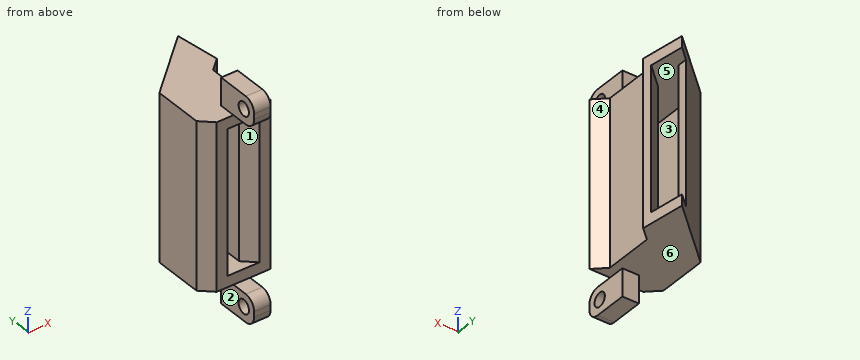
```python
from build123d import *

# Parameters (mm, degrees)
PAD007_DEPTH    = 30
SKETCH021_W     = 5.75
SKETCH021_H     = 26
SKETCH023_W     = 2.875
SKETCH023_H     = 26
POCKET009_DEPTH = 5
SKETCH024_W     = 3
SKETCH024_H     = 3
PAD008_DEPTH    = 5
PAD008_FACE6_W  = 3
PAD008_FACE6_H  = 5
PAD009_DEPTH    = 5
SKETCH025_W     = 3
SKETCH025_H     = 3
PAD010_DEPTH    = 5
PAD010_FACE7_W  = 3
PAD010_FACE7_H  = 5
PAD011_DEPTH    = 5
SKETCH026_R     = 1.25
POCKET010_DEPTH = 5
FILLET_R        = 2


with BuildPart() as part:
    # Sketch020 → Pad007 (new body)
    with BuildSketch(Plane.XY):
        Polygon((-9.75, -21), (-11.9217087917, -19), (-11.9217087917, -10), (-1.063164833, 0), (0, -8), (-2.1717087917, -10), (-2.1717087917, -19), (0, -21), align=None)
    extrude(amount=PAD007_DEPTH)

    # SubtractivePipe: sweep along a path in Sketch022
    with BuildLine(Plane.XY.offset(30)) as subtractivepipe_path:
        Line((-4.875, -21), (-7.0467087917, -19))
        Line((-7.0467087917, -19), (-7.0467087917, -10))
        Line((-7.0467087917, -10), (-0.5315824165, -4))
    # Sketch021 (on Face8 of Pad007) → SubtractivePipe (sweep, cut)
    with BuildSketch(Plane.XZ.offset(21)):
        with Locations((-4.875, 15)):
            Rectangle(SKETCH021_W, SKETCH021_H)
    sweep(path=subtractivepipe_path.line, mode=Mode.SUBTRACT)

    # Sketch023 (on Face22 of SubtractivePipe) → Pocket009 (cut)
    with BuildSketch(Plane.XZ.offset(4)):
        with Locations((-1.9690824165, 15)):
            Rectangle(SKETCH023_W, SKETCH023_H)
    extrude(amount=-POCKET009_DEPTH, mode=Mode.SUBTRACT)

    # Sketch024 (on Face4 of Pocket009) → Pad008 (join)
    with BuildSketch(Plane(origin=(0, 0, 0), x_dir=(1, 0, 0), z_dir=(0, 0, -1))):
        with Locations((-5.2, 19.5)):
            Rectangle(SKETCH024_W, SKETCH024_H)
    extrude(amount=PAD008_DEPTH)

    # Pad008 Face6 → Pad009 (add)
    with BuildSketch(Plane(origin=(-5.2, -21, -2.5), x_dir=(-1, 0, 0), z_dir=(0, -1, 0))):
        Rectangle(PAD008_FACE6_W, PAD008_FACE6_H)
    extrude(amount=PAD009_DEPTH)

    # Sketch025 (on Face5 of Pad009) → Pad010 (join)
    with BuildSketch(Plane.XY.offset(30)):
        with Locations((-5.2, -19.5)):
            Rectangle(SKETCH025_W, SKETCH025_H)
    extrude(amount=PAD010_DEPTH)

    # Pad010 Face7 → Pad011 (add)
    with BuildSketch(Plane(origin=(-5.2, -21, 32.5), x_dir=(-1, 0, 0), z_dir=(0, -1, 0))):
        Rectangle(PAD010_FACE7_W, PAD010_FACE7_H)
    extrude(amount=PAD011_DEPTH)

    # Sketch026 → Pocket010 (cut)
    with BuildSketch(Plane(origin=(-6.7, 0, 0), x_dir=(0, -1, 0), z_dir=(-1, 0, 0))):
        with Locations((23.5, -2.5)):
            Circle(SKETCH026_R)
        with Locations((23.5, 32.5)):
            Circle(SKETCH026_R)
    extrude(amount=-POCKET010_DEPTH, mode=Mode.SUBTRACT)

    # Fillet
    fillet_edges = [part.edges().sort_by_distance(p)[0] for p in [
        (-5.2, -26, 35),
        (-5.2, -26, 30),
        (-5.2, -26, 0),
        (-5.2, -26, -5),
    ]]
    fillet(fillet_edges, radius=FILLET_R)


with BuildPart() as part_1:
    # Body002 placement: moved
    add(part.part.moved(Location((-0.2, 61.7, -30.6))))


solid = part_1.part
```
The listing builds one solid part. Answer for the finished solid, in the listing's coordinates (mm). Face numbers are marked on the shaded views. A direction names the side the tool comes from. Give positions to 0.01 mm unless a question says otherwise; leave off trailing zeros. Loops run counter-clockwise (first coordinate to the right, second up) from the corner with the lowest first, then second, coordinate; pieces in that order, holes last. Notation, with made-up numbers: M -2,76.5 L 16,76.5 A20 cw 16,106.5 Z; hole C -22.5,21.5 d6. An arc over 180 degrees is marked long. One line per item, written item: value.
1. For a pull along X with two mould halves and no side action, classify the marked faces 4, 5 and 6 as pulls with the +X half, pulls with the -X half, needs draft (parallel to the pull), parting line crosses it, or undercut.
Found:
face 4: pulls with the +X half
face 5: undercut
face 6: needs draft
2. Section A-A on z = -33.1 is taken. Determine the outline of the cut face in (x, y).
Found:
outline: M -6.9,35.7 L -3.9,35.7 L -3.9,36.95 L -6.9,36.95 Z; M -6.9,39.45 L -3.9,39.45 L -3.9,43.7 L -6.9,43.7 Z
3. For the marked faces 1, 2 and 3, determine the directions among +Z, -Z, +X, -X, +Y, -Y from which every point of the face is accessible in a straight line to the end or side of a thin tool.
Found:
face 1: -Y
face 2: -Z, -X, +Y, -Y
face 3: none
4. Section B-B on y = 44.75 is taken. Determine the outline of the cut face in (x, z), plus the area to 3 significant figures.
Found:
outline: M -12.12,-30.6 L -2.37,-30.6 L -2.37,-0.6 L -12.12,-0.6 Z; hole M -10.12,-28.6 L -4.37,-28.6 L -4.37,-2.6 L -10.12,-2.6 Z
area: 143 mm^2
5. Find the intervals of material crossed by probe 1 along Z at (x, y) = (-4.6, 38.2); probe 2 along X at (y, z) = (50, -9.5); probe 3 along Z at (x, y) = (-1.5, 57.25), in increasing order.
Found:
probe 1: -35.6 to -34.35, -31.85 to -30.6, -0.6 to 0.65, 3.15 to 4.4
probe 2: -12.12 to -10.12, -4.37 to -2.37
probe 3: -30.6 to -28.6, -2.6 to -0.6
6. Each of these flat-tipped pins is pushed along its axis until it touches: P1, Ø1.5, axis at y = 38, z = 3, coming from the +X side; P2, Ø6, axis at x = -7, y = 49, coming from the +Z side; P3, Ø3, axis at x = -7, y = 54.5, coming from the -Z side. Where does it stop, or does it pass through?
Found:
P1: x = -3.9
P2: z = -0.6
P3: z = -30.6
7. Section C-C on y = 38.2 is taken. Determine the outline of the cut face in (x, z).
Found:
outline: M -6.9,-35.6 L -3.9,-35.6 L -3.9,-34.35 L -6.9,-34.35 Z; M -6.9,-31.85 L -3.9,-31.85 L -3.9,-30.6 L -6.9,-30.6 Z; M -6.9,-0.6 L -3.9,-0.6 L -3.9,0.65 L -6.9,0.65 Z; M -6.9,3.15 L -3.9,3.15 L -3.9,4.4 L -6.9,4.4 Z
8. Section D-D on x = -8.5 is taken. Determine the outline of the cut face in (y, z), plus the area to 3 significant figures.
Found:
outline: M 40.7,-30.6 L 55.04,-30.6 L 55.04,-0.6 L 40.7,-0.6 Z; hole M 41.21,-28.6 L 53.19,-28.6 L 53.19,-2.6 L 41.21,-2.6 Z
area: 118 mm^2
